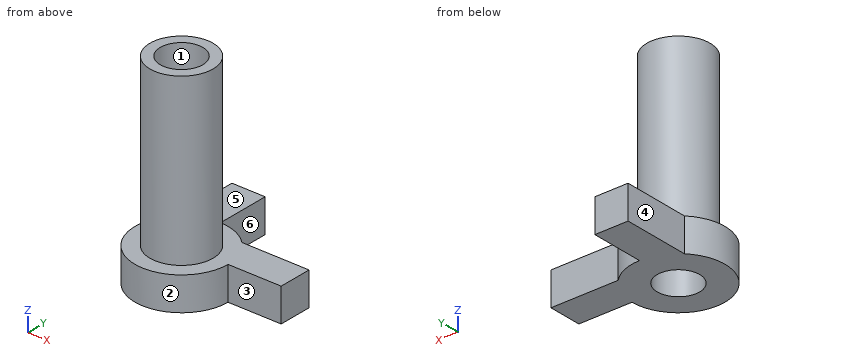
```python
from build123d import *

# Parameters (mm, degrees)
CYLINDER_R             = 3.2
CYLINDER_DEPTH         = 30
BOX001_W               = 15
BOX001_H               = 5
BOX001_DEPTH           = 5
BOX001_PLACEMENT_ANGLE = 90
BOX_W                  = 15
BOX_H                  = 5
BOX_DEPTH              = 5
CYLINDER001_R          = 4.75
CYLINDER001_DEPTH      = 30
CYLINDER002_R          = 7
CYLINDER002_DEPTH      = 5


with BuildPart() as cylinder:
    # Cylinder → Cylinder (new body)
    with BuildSketch(Plane.XY):
        Circle(CYLINDER_R)
    extrude(amount=CYLINDER_DEPTH)


with BuildPart() as box001:
    # Box001 → Box001 (new body)
    with BuildSketch(Plane.XY):
        with Locations((7.5, 2.5)):
            Rectangle(BOX001_W, BOX001_H)
    extrude(amount=BOX001_DEPTH)


with BuildPart() as box001_1:
    # Box001 placement: moved
    add(box001.part.rotate(Axis((0, 0, 0), (0, 0, 1)), BOX001_PLACEMENT_ANGLE))


with BuildPart() as box:
    # Box → Box (new body)
    with BuildSketch(Plane.XY):
        with Locations((7.5, 2.5)):
            Rectangle(BOX_W, BOX_H)
    extrude(amount=BOX_DEPTH)


with BuildPart() as cylinder001:
    # Cylinder001 → Cylinder001 (new body)
    with BuildSketch(Plane.XY):
        Circle(CYLINDER001_R)
    extrude(amount=CYLINDER001_DEPTH)


with BuildPart() as cut:
    # Cylinder002 → Cylinder002 (new body)
    with BuildSketch(Plane.XY):
        Circle(CYLINDER002_R)
    extrude(amount=CYLINDER002_DEPTH)

    # Fusion: union Cylinder001
    add(cylinder001.part)

    # Fusion001: union Box001, Box
    add(box001_1.part)
    add(box.part)

    # Cut: cut Cylinder
    add(cylinder.part, mode=Mode.SUBTRACT)


solid = cut.part
```
Check sheet for the modelled part. Datum: model origin and axes. Units: mm. Face numbers are marked on the shaded views. A direction names the side the tool comes from. Coordinates: 2 decimals unless noted, no trailing zeros. Order: outer loops, then holes, each group sorted by start corner. A loop starts at its lowest first (then second) coordinate and runs counter-clockwise, first axis right, second up. Notation, with made-up numbers: (30, 74.5) -> (85, 74.5) arc R23 ccw to (85, 106.5) -> close; hole circle Ø1 at (0.5, 32.5). An arc over 180 degrees is marked (long way). Write each question's results on one line, items separated by ' | '. Start each with the question number.
1) Section check A-A (x = 2.5). Enter the section's corners in (y, z), and give its area (3 significant figures).
2) Section check B-B (z = 7). Enter the section's corners in (x, y).
3) Set-up check for the marked faces 4, 5 and 6: record each of +Z, -Z, +X, -X, +Y, -Y from which the full face is reachable in a straight line by a thin tool's end or side.
4) Depth check by flat-ended pin: pin 1 (6 mm diameter, centred on x = 9.5, y = 6, fed in from +Z); pin 2 (2.5 mm diameter, centred on x = 12.5, z = 3, fed in from -Y); pin 3 (10 mm diameter, centred on x = 11, z = 4, fed in from -Y). Enter the tip coordinate at first touch or a pass-through.
5) Draft check along X on the marked faces 1, 2 and 3. Enter one of: pulls with the +X half, pulls with the -X half, needs draft (parallel to the pull), parting line crosses it, or undercut.
6) Section check D-D (y = 11). Enter the section's corners in (x, z), and give its area (3 significant figures).
7) Material ranges on line 1 along Y through (x, z) = (0, 20); line 2 along Z through (x, y) = (-4.5, -4.75); line 3 along X through (y, z) = (-0.5, 12.5), recorded low to high.
8) Section check C-C (y = 1). Enter the section's corners in (x, z).
Checked values:
1) outline: (-6.54, 0) -> (-2, 0) -> (-2, 30) -> (-4.04, 30) -> (-4.04, 5) -> (-6.54, 5) -> close; (2, 0) -> (6.54, 0) -> (6.54, 5) -> (4.04, 5) -> (4.04, 30) -> (2, 30) -> close | area: 147 mm²
2) outline: circle Ø9.5 at (0, 0); hole circle Ø6.4 at (0, 0)
3) face 4: +Z, -Z, -X, +Y | face 5: +Z | face 6: +Z, -Z, +X, +Y
4) pin 1: z = 5 | pin 2: y = 0 | pin 3: y = -3.61
5) face 1: undercut | face 2: parting line crosses it | face 3: needs draft
6) outline: (-5, 0) -> (0, 0) -> (0, 5) -> (-5, 5) -> close | area: 25.0 mm²
7) line 1: -4.75 to -3.2, 3.2 to 4.75 | line 2: 0 to 5 | line 3: -4.72 to -3.16, 3.16 to 4.72
8) outline: (-6.93, 0) -> (-3.04, 0) -> (-3.04, 30) -> (-4.64, 30) -> (-4.64, 5) -> (-6.93, 5) -> close; (3.04, 0) -> (15, 0) -> (15, 5) -> (4.64, 5) -> (4.64, 30) -> (3.04, 30) -> close
